Study the drawing (mm; zero at the part's minimum x, y, z) and answer. Round coordinates to 2 decimals unless told otherwise and drop trailing zeros. Loops run counter-clockwise (first coordinate to the right, second up) from the corner with the lowest first, then second, coordinate; pieces in that order, holes last. Notation, with made-up numbers: (-22.75, -5) -> (-5.75, -5) arc R14 ccw to (-5.75, 17) -> close; hole circle Ø9 at (-27.75, -15.75). An arc over 180 degrees is marked (long way). Write each question's results on one line, items separated by ' | '. Start each with the question number.
(1) The part is cut by section B-B (y = 0.75). Determine the outline of the cut face in (x, z).
(2) Straight lines are drawn through the part: probe 1 along X at (y, z) = (5.75, 0.25); probe 2 along Y at (x, z) = (7.25, 0.15). For each, find the intervals that lie inside material, in ascending order.
(3) The part is cut by section C-C (x = 7). Determine the outline of the cut face in (y, z).
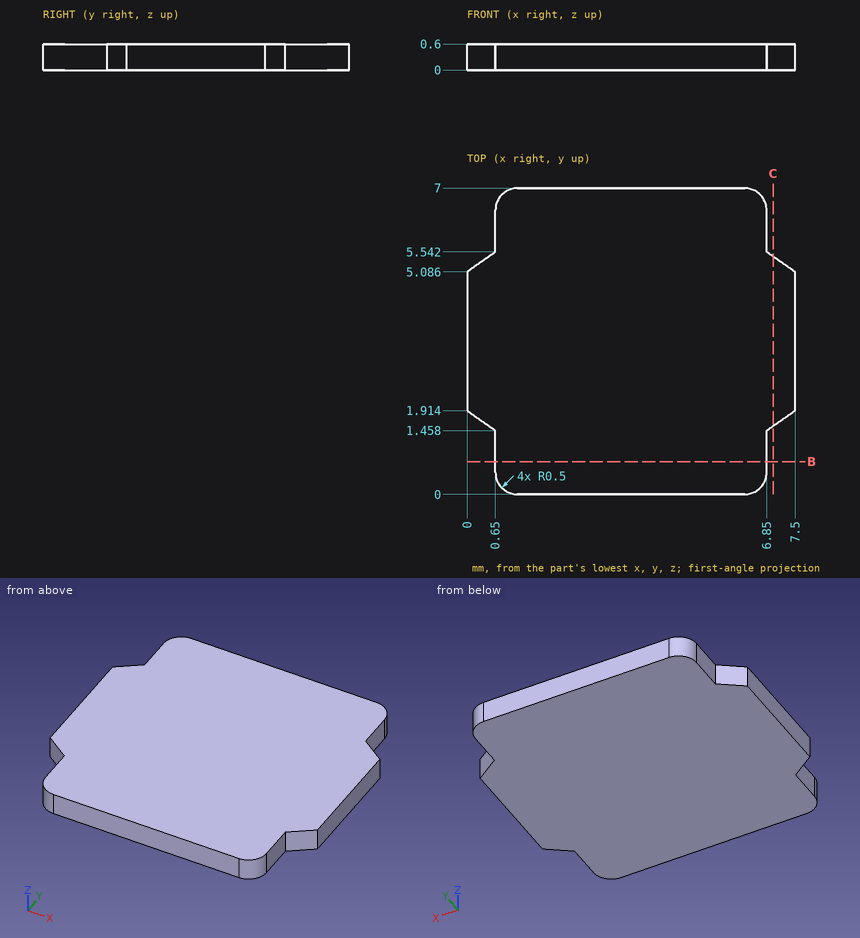
Checked values:
1) outline: (0.65, 0) -> (6.85, 0) -> (6.85, 0.6) -> (0.65, 0.6) -> close
2) probe 1: x = 0.65 to 6.85 | probe 2: y = 1.74 to 5.26
3) outline: (1.56, 0) -> (5.44, 0) -> (5.44, 0.6) -> (1.56, 0.6) -> close
